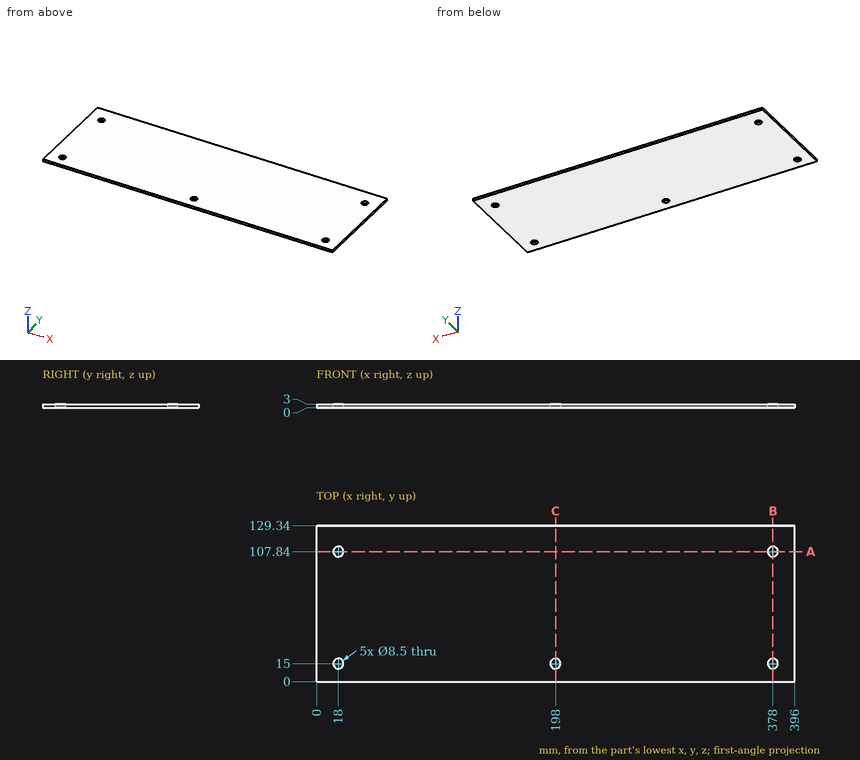
Can you work these out from the drawing? Everything is in mm from the part's minimum corner. Coordinates: 2 decimals unless noted, no trailing zeros. Write each loop counter-clockwise with the first axis right and the second up, starting at its lowest first coordinate (ties: lowest second). Pieces come first, ordered by that corner, then holes. Notation, with made-up numbers: (50.25, -22.5) -> (97.25, -22.5) arc R27 ccw to (97.25, 14.5) -> close; hole circle Ø3 at (73.5, 0). An arc over 180 degrees is marked (long way). Write each question's results on one line, items separated by ' | '. Start each with the question number.
Q1. Imagine slicing it at A-A (y = 107.84). Write out the boundary of the cut face in (x, z).
Q2. Imagine slicing it at B-B (x = 378). Write out the boundary of the cut face in (y, z), then the cut area to 3 significant figures.
Q3. If I drill on probe 1 along Y at (x, z) = (378, 1.2); probe 2 along Y at (x, z) = (198, 2.05), over which ranges is the centre line in solid material (lowest first)?
Q4. I'm going to push flat-ended pins straight in: pin 1 (7 mm diameter, centred on x = 378, y = 107.84, fed in from -Z); pin 2 (10 mm diameter, centred on x = 280, y = 113, fed in from -Z). Where does each tip first touch, or does it pass through?
Q5. Imagine slicing it at C-C (x = 198). Write out the boundary of the cut face in (y, z), then the cut area to 3 significant figures.
Taken from the geometry:
1) outline: (0, 0) -> (13.75, 0) -> (13.75, 3) -> (0, 3) -> close; (22.25, 0) -> (373.75, 0) -> (373.75, 3) -> (22.25, 3) -> close; (382.25, 0) -> (396, 0) -> (396, 3) -> (382.25, 3) -> close
2) outline: (0, 0) -> (10.75, 0) -> (10.75, 3) -> (0, 3) -> close; (19.25, 0) -> (103.59, 0) -> (103.59, 3) -> (19.25, 3) -> close; (112.09, 0) -> (129.34, 0) -> (129.34, 3) -> (112.09, 3) -> close | area: 337 mm^2
3) probe 1: y = 0 to 10.75, 19.25 to 103.59, 112.09 to 129.34 | probe 2: y = 0 to 10.75, 19.25 to 129.34
4) pin 1: passes through | pin 2: stops at z = 0
5) outline: (0, 0) -> (10.75, 0) -> (10.75, 3) -> (0, 3) -> close; (19.25, 0) -> (129.34, 0) -> (129.34, 3) -> (19.25, 3) -> close | area: 363 mm^2
